from build123d import *

# Parameters (mm, degrees)
EXTRUDE_1_DEPTH     = 3
FILLET_1_R          = 5
FILLET_2_R          = 10
FILLET_3_R          = 3
SKETCH_2_R          = 1.6
CUT_EXTRUDE_1_DEPTH = 3
FILLET_4_R          = 3


with BuildPart() as part:
    # 草图1 → 凸台-拉伸1 (new body)
    with BuildSketch(Plane.XY):
        Polygon((0, -15), (-15.87797303, -15), (-0.208100049, -42.141016151), (-13.198481106, -49.641016151), (-80, -15), (-80, 0), (0, 0), align=None)
        Polygon((-17.839906221, -41.601832032), (-33.198481106, -15), (-69.138712739, -15), align=None, mode=Mode.SUBTRACT)
    extrude(amount=EXTRUDE_1_DEPTH)

    # 圆角1
    fillet_1_edges = [part.edges().sort_by_distance(p)[0] for p in [
        (-15.87797303, -15, 1.5),
    ]]
    fillet(fillet_1_edges, radius=FILLET_1_R)

    # 圆角2
    fillet_2_edges = [part.edges().sort_by_distance(p)[0] for p in [
        (-33.198481106, -15, 1.5),
    ]]
    fillet(fillet_2_edges, radius=FILLET_2_R)

    # 圆角3
    fillet_3_edges = [part.edges().sort_by_distance(p)[0] for p in [
        (0, -15, 1.5),
        (-0.208100049, -42.141016151, 1.5),
        (-13.198481106, -49.641016151, 1.5),
        (-80, -15, 1.5),
        (-80, 0, 1.5),
        (0, 0, 1.5),
    ]]
    fillet(fillet_3_edges, radius=FILLET_3_R)

    # 草图2 → 切除-拉伸1 (cut)
    with BuildSketch(Plane.XY.offset(3)):
        with Locations((-11.703290577, -37.230762114)):
            Circle(SKETCH_2_R)
        with Locations((-19.203290577, -24.240381057)):
            Circle(SKETCH_2_R)
        with Locations((-10, -7.5)):
            Circle(SKETCH_2_R)
        with Locations((-25, -7.5)):
            Circle(SKETCH_2_R)
        with Locations((-40, -7.5)):
            Circle(SKETCH_2_R)
        with Locations((-55, -7.5)):
            Circle(SKETCH_2_R)
        with Locations((-70, -7.5)):
            Circle(SKETCH_2_R)
    extrude(amount=-CUT_EXTRUDE_1_DEPTH, mode=Mode.SUBTRACT)

    # 圆角4
    fillet_4_edges = [part.edges().sort_by_distance(p)[0] for p in [
        (-69.138712739, -15, 1.5),
        (-17.839906221, -41.601832032, 1.5),
    ]]
    fillet(fillet_4_edges, radius=FILLET_4_R)


solid = part.part
Work out the finished part from the listing and answer in its coordinate system (mm). A direction names the side the tool comes from. Give positions to 0.01 mm unless a question says otherwise; leave off trailing zeros. Loops run counter-clockwise (first coordinate to the right, second up) from the corner with the lowest first, then second, coordinate; pieces in that order, holes last. Notation, with made-up numbers: (-3.5, 70.5) - (23.5, 70.5) arc R19 ccw to (23.5, 76.5) - close; hole circle Ø6 at (-5.5, 28.5). An arc over 180 degrees is marked (long way). Answer in a Markdown table with one row per item.
(1) Section A-A (y = -7.5) is taken. Give the vertices of the cut face in (x, z), and give its area (3 significant figures).
Results list:
| item | result |
|---|---|
| outline | (-80, 0) - (-71.6, 0) - (-71.6, 3) - (-80, 3) - close; (-68.4, 0) - (-56.6, 0) - (-56.6, 3) - (-68.4, 3) - close; (-53.4, 0) - (-41.6, 0) - (-41.6, 3) - (-53.4, 3) - close; (-38.4, 0) - (-26.6, 0) - (-26.6, 3) - (-38.4, 3) - close; (-23.4, 0) - (-11.6, 0) - (-11.6, 3) - (-23.4, 3) - close; (-8.4, 0) - (0, 0) - (0, 3) - (-8.4, 3) - close |
| area | 192 mm² |
(2) Flat-ended cylindrical pins translate along their axes: pin 1 Ø4 at (x, y) = (-25, -7.5) entering from -Z; pin 2 Ø1 at (x, z) = (-17.5, 2) entering from -Y; pin 3 Ø3 at (x, y) = (-11.7, -37.23) entering from -Z; pin 4 Ø1.5 at (x, z) = (-5, 1.5) entering from -Y. Find the tip coordinate at first contact, or state that the pin passes through.
Results list:
| item | result |
|---|---|
| pin 1 | stops at z = 0 |
| pin 2 | stops at y = -47.67 |
| pin 3 | passes through |
| pin 4 | stops at y = -45.34 |
(3) For a pull along X with two mould halves and no side action, classify faces 4 (the face through (-68.474, -7.019, 1.521)), 5 (the face through (-53.52, -8.11, 1.52)), 6 (the face through (-7.228, -46.194, 1.479)), 7 (the face through (-30.6, -18.8, 0)) as pulls with the +X half, pulls with the -X half, needs draft (parallel to the pull), parting line crosses it, or undercut.
Results list:
| item | result |
|---|---|
| face 4 | undercut |
| face 5 | undercut |
| face 6 | pulls with the +X half |
| face 7 | needs draft |
(4) A tool of negligible diameter and unlimited length cuts with its end or side. For faces 1 (the face through (-48, -15, 1)), 2 (the face through (-6.7, -30.9, 1.5)), 3 (the face through (0, -7, 1)), from which of +Z, -Z, +X, -X, +Y, -Y can it reach the whole face along a straight path? Write none if from no direction.
Results list:
| item | result |
|---|---|
| face 1 | +Z, -Z |
| face 2 | +Z, -Z, +X |
| face 3 | +Z, -Z, +X, +Y, -Y |
(5) Section D-D (x = -32.5) is taken. Give the vertices of the cut face in (y, z).
Results list:
| item | result |
|---|---|
| outline | (-39.63, 0) - (-34, 0) - (-34, 3) - (-39.63, 3) - close; (-17.38, 0) - (0, 0) - (0, 3) - (-17.38, 3) - close |
(6) Section C-C (z = 2.45) is taken. State how many separate pieces and enclosed holes the cut face has, and give its area (3 significant figures).
Results list:
| item | result |
|---|---|
| separate pieces | 1 |
| enclosed holes | 8 |
| area | 2,070 mm² |
(7) Consider L1, parallel to X at y = -25, z = 1.4; L2, parallel to Y at x = -55, z = 1.2; L3, parallel to Y at x = -40, z = 1.95. Determine where each line is inside the solid, lowest interval first. Write a range as [from, to].
Results list:
| item | result |
|---|---|
| L1 | x = [-60.72, -49.85], [-27.42, -20.61], [-17.8, -10.1] |
| L2 | y = [-27.96, -22.33], [-15, -9.1], [-5.9, 0] |
| L3 | y = [-35.74, -30.11], [-15, -9.1], [-5.9, 0] |
(8) Section B-B (x = -24.5) is taken. Give the vertices of the cut face in (y, z), and give its area (3 significant figures).
Results list:
| item | result |
|---|---|
| outline | (-43.78, 0) - (-37.02, 0) - (-37.02, 3) - (-43.78, 3) - close; (-30.07, 0) - (-9.02, 0) - (-9.02, 3) - (-30.07, 3) - close; (-5.98, 0) - (0, 0) - (0, 3) - (-5.98, 3) - close |
| area | 101 mm² |
